from build123d import *

# Parameters (mm, degrees)
F0_W          = 80
F0_H          = 25
F1_DEPTH      = 40
F2_W          = 3
F2_H          = 20
F3_DEPTH      = 15
F4_R          = 7
F5_R          = 7
F7_D          = 5
F9_D          = 5
F10_T         = 3
F10_T3_DEPTH  = 21
F10_T5_DEPTH  = 9
F10_T7_DEPTH  = 9
F10_T9_DEPTH  = 9
F10_T11_DEPTH = 9
F10_T13_DEPTH = 9


# Not quite as in the source:
# - a shell that OpenCascade refuses in one call is made with other operations: the cavity is built on its own and cut out


with BuildPart() as f1:
    # F0 (on Top) → F1 (new body)
    with BuildSketch(Plane.XY):
        Rectangle(F0_W, F0_H)
    extrude(amount=F1_DEPTH)

    # F2 (on face) → F3 (join)
    with BuildSketch(Plane(origin=(0, 0, 0), x_dir=(1, 0, 0), z_dir=(0, 0, -1))):
        with Locations((-6, 22.5)):
            Rectangle(F2_W, F2_H)
        with Locations((0, 22.5)):
            Rectangle(F2_W, F2_H)
        with Locations((6, 22.5)):
            Rectangle(F2_W, F2_H)
        with Locations((3, -22.5)):
            Rectangle(F2_W, F2_H)
        with Locations((-3, -22.5)):
            Rectangle(F2_W, F2_H)
    extrude(amount=-F3_DEPTH)

    # F4
    f4_edges = [f1.edges().sort_by_distance(p)[0] for p in [
        (3, 32.5, 0),
        (-3, 32.5, 0),
        (-3, 32.5, 15),
        (3, 32.5, 15),
    ]]
    fillet(f4_edges, radius=F4_R)

    # F5
    f5_edges = [f1.edges().sort_by_distance(p)[0] for p in [
        (-6, -32.5, 15),
        (0, -32.5, 15),
        (6, -32.5, 15),
        (6, -32.5, 0),
        (0, -32.5, 0),
        (-6, -32.5, 0),
    ]]
    fillet(f5_edges, radius=F5_R)

    # F7 (through all)
    with Locations(Plane(origin=(-7.5, 0, 0), x_dir=(0, -1, 0), z_dir=(-1, 0, 0))):
        with Locations((25, 7.5)):
            Hole(F7_D / 2)

    # F9 (through all)
    with Locations(Plane(origin=(-4.5, 0, 0), x_dir=(0, -1, 0), z_dir=(-1, 0, 0))):
        with Locations((-23.3794022352, 7.5034750625)):
            Hole(F9_D / 2)

    # F10: shell of thickness 3, made by hand


with BuildPart() as f10_core1:
    # F10_t2: copy of F1
    add(f1.part)

    # the walls: a layer under each face that stays
    f10_faces = [f10_core1.faces().sort_by_distance(p)[0] for p in [
        (0, 0, 0),
        (7.5, -15.8333333333, 12.5),
        (6, -30.4497474683, 2.0502525317),
        (0, -12.5, 20),
        (4.5, -29.1666666667, 12.5),
        (40, 0, 20),
        (0, 12.5, 20),
        (1.5, -15.8333333333, 12.5),
        (4.5, 29.1666666667, 12.5),
        (0, -30.4497474683, 2.0502525317),
        (3, 30.4497474683, 2.0502525317),
        (-1.5, -29.1666666667, 12.5),
        (1.5, 15.8333333333, 12.5),
        (-4.5, -15.8333333333, 12.5),
        (-1.5, 29.1666666667, 12.5),
        (-6, -30.4497474683, 2.0502525317),
        (-3, 30.4497474683, 2.0502525317),
        (-7.5, -29.1666666667, 12.5),
        (-4.5, 15.8333333333, 12.5),
        (-40, 0, 20),
        (6, -32.5, 7.5),
        (6, -30.4497474683, 12.9497474683),
        (6, -19, 15),
        (6, -22.5, 7.5),
        (-6, -19, 15),
        (0, -19, 15),
        (3, 19, 15),
        (-3, 19, 15),
        (0, -32.5, 7.5),
        (0, -30.4497474683, 12.9497474683),
        (0, -22.5, 7.5),
        (3, 32.5, 7.5),
        (3, 30.4497474683, 12.9497474683),
        (3, 25.8794022352, 7.5034750625),
        (-6, -32.5, 7.5),
        (-6, -30.4497474683, 12.9497474683),
        (-6, -22.5, 7.5),
        (-3, 32.5, 7.5),
        (-3, 30.4497474683, 12.9497474683),
        (-3, 25.8794022352, 7.5034750625),
    ]]
    thicken(f10_faces, amount=-F10_T, mode=Mode.SUBTRACT)

    # F10_s4 → F10_t3 (cut)
    with BuildSketch(Plane.XY.offset(-3)):
        Polygon((7.53, -12.53), (4.5, -12.5), (4.5, -9.5), (7.5, -9.5), align=None)
        Polygon((-7.53, -12.53), (-7.5, -9.5), (-4.5, -9.5), (-4.5, -12.5), align=None)
        Polygon((-4.47, -12.53), (-4.5, -9.5), (-7.5, -9.5), (-7.5, -12.5), align=None)
        Polygon((-1.53, -12.53), (-1.5, -9.5), (1.5, -9.5), (1.5, -12.5), align=None)
        Polygon((1.53, -12.53), (1.5, -9.5), (-1.5, -9.5), (-1.5, -12.5), align=None)
        Polygon((4.47, -12.53), (4.5, -9.5), (7.5, -9.5), (7.5, -12.5), align=None)
        Polygon((4.53, 12.53), (4.5, 9.5), (1.5, 9.5), (1.5, 12.5), align=None)
        Polygon((1.47, 12.53), (1.5, 9.5), (4.5, 9.5), (4.5, 12.5), align=None)
        Polygon((-1.47, 12.53), (-1.5, 9.5), (-4.5, 9.5), (-4.5, 12.5), align=None)
        Polygon((-4.53, 12.53), (-4.5, 9.5), (-1.5, 9.5), (-1.5, 12.5), align=None)
    extrude(amount=F10_T3_DEPTH, mode=Mode.SUBTRACT)

    # F10_s6 → F10_t5 (cut)
    with BuildSketch(Plane.YZ.offset(-10.5)):
        Polygon((-12.53, 15.03), (-9.5, 15), (-9.5, 12), (-12.5, 12), align=None)
    extrude(amount=F10_T5_DEPTH, mode=Mode.SUBTRACT)

    # F10_s8 → F10_t7 (cut)
    with BuildSketch(Plane.YZ.offset(-4.5)):
        Polygon((-12.53, 15.03), (-9.5, 15), (-9.5, 12), (-12.5, 12), align=None)
    extrude(amount=F10_T7_DEPTH, mode=Mode.SUBTRACT)

    # F10_s10 → F10_t9 (cut)
    with BuildSketch(Plane.YZ.offset(1.5)):
        Polygon((-12.53, 15.03), (-9.5, 15), (-9.5, 12), (-12.5, 12), align=None)
    extrude(amount=F10_T9_DEPTH, mode=Mode.SUBTRACT)

    # F10_s12 → F10_t11 (cut)
    with BuildSketch(Plane.YZ.offset(-1.5)):
        Polygon((12.53, 15.03), (9.5, 15), (9.5, 12), (12.5, 12), align=None)
    extrude(amount=F10_T11_DEPTH, mode=Mode.SUBTRACT)

    # F10_s14 → F10_t13 (cut)
    with BuildSketch(Plane.YZ.offset(-7.5)):
        Polygon((12.53, 15.03), (9.5, 15), (9.5, 12), (12.5, 12), align=None)
    extrude(amount=F10_T13_DEPTH, mode=Mode.SUBTRACT)


with BuildPart() as f1_1:
    add(f1.part)

    # what is left inside the walls is the cavity
    f10_cavity = [f10_core1.part.solids().sort_by_distance(p)[0] for p in [
        (0, 9.47, 27.666667),
    ]]
    add(f10_cavity, mode=Mode.SUBTRACT)


solid = f1_1.part
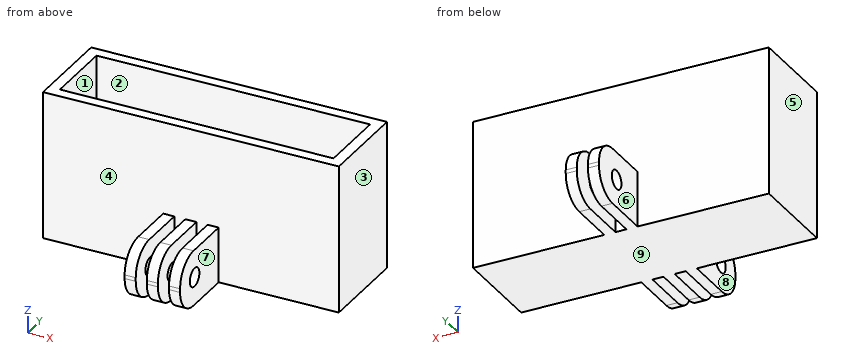
The model under review builds one solid part; all positions refer to its coordinate system, in mm. Face numbers are marked on the shaded views. A direction names the side the tool comes from. Coordinates: 2 decimals unless noted, no trailing zeros. Write each loop counter-clockwise with the first axis right and the second up, starting at its lowest first coordinate (ties: lowest second). Pieces come first, ordered by that corner, then holes. Notation, with made-up numbers: (-26.75, -16) - (32.25, -16) arc R13 cw to (32.25, 9) - close; hole circle Ø4 at (49, 74.25). An arc over 180 degrees is marked (long way). Answer as CSV lines item,"result".
(1) We need section C-C (y = -15). Give the boundary of the cut face in (x, z).
Data:
outline,"(-7.5, 0) - (-4.5, 0) - (-4.5, 15) - (-7.5, 15) - close; (-1.5, 0) - (1.5, 0) - (1.5, 15) - (-1.5, 15) - close; (4.5, 0) - (7.5, 0) - (7.5, 15) - (4.5, 15) - close"
(2) Clearance check with flat-ended pins moving along their axes: pin 1 Ø4.5 at (y, z) = (19.5, 9) entering from +X; pin 2 Ø2 at (y, z) = (22.5, 5) entering from -X; pin 3 Ø4.5 at (y, z) = (23.38, 7.5) entering from -X; pin 4 Ø8 at (y, z) = (-25, 7.5) entering from -X. State where each tip first meets the part, or that it passes through.
Data:
pin 1,"stops at x = 4.5"
pin 2,"stops at x = -4.5"
pin 3,"passes through"
pin 4,"stops at x = -7.5"
(3) For line 1 along Z through (x, y) = (0, -25); line 2 along Y through (x, z) = (-6, 32.5); line 3 along X through (y, z) = (-0.5, 23), list the stretches that pass through material, from the lowest coordinate up. Write a range as [from, to].
Data:
line 1,"z = [0, 5], [10, 15]"
line 2,"y = [-12.5, -9.5], [9.5, 12.5]"
line 3,"x = [-40, -37], [37, 40]"
(4) Mouldability with a two-part tool opening along Y and no side actions: class the marked faces 1, 2, 3 and 4 as pulls with the +Y half, pulls with the -Y half, needs draft (parallel to the pull), parting line crosses it, or undercut.
Data:
face 1,"undercut"
face 2,"undercut"
face 3,"needs draft"
face 4,"pulls with the -Y half"
(5) We need section A-A (y = 19). Give the boundary of the cut face in (x, z), plus the area to 3 significant figures.
Data:
outline,"(-4.5, 0) - (-1.5, 0) - (-1.5, 15) - (-4.5, 15) - close; (1.5, 0) - (4.5, 0) - (4.5, 15) - (1.5, 15) - close"
area,"90.0 mm2"
(6) Tool access review of the marked faces 5, 6, 7, 8 and 9: name each direction out of +Z, -Z, +X, -X, +Y, -Y from which nothing blocks a thin tool from reaching the whole face with its end or side.
Data:
face 5,"+Z, -Z, -X, +Y, -Y"
face 6,"+Z, -Z, -X, +Y"
face 7,"+Z, -Z, +X, -Y"
face 8,"+Z, -Z, -X, -Y"
face 9,"-Z, +X, -X, +Y, -Y"
(7) We need section D-D (x = 12.5). Give the boundary of the cut face in (y, z), plus the area to 3 significant figures.
Data:
outline,"(-12.5, 0) - (12.5, 0) - (12.5, 40) - (9.5, 40) - (9.5, 3) - (-9.5, 3) - (-9.5, 40) - (-12.5, 40) - close"
area,"297 mm2"
(8) We need section B-B (z = 28). Give the boundary of the cut face in (x, y), plus the area to 3 significant figures.
Data:
outline,"(-40, -12.5) - (40, -12.5) - (40, 12.5) - (-40, 12.5) - close; hole (-37, -9.5) - (37, -9.5) - (37, 9.5) - (-37, 9.5) - close"
area,"594 mm2"
